Check sheet for the drawn part. Datum: minimum x, y, z corner. Units: mm. A direction names the side the tool comes from. Give positions to 0.01 mm unless a question says otherwise; leave off trailing zeros. Write each loop counter-clockwise with the first axis right and the second up, starting at its lowest first coordinate (ties: lowest second). Pieces come first, ordered by that corner, then holes. Notation, with made-up numbers: (87.5, 9.25) - (114.5, 9.25) arc R14 cw to (114.5, 26.25) - close; hole circle Ø3 at (49.25, 67.5). An arc over 180 degrees is marked (long way). One line per question, with ' | ' between items. Start each with the question number.
Q1. Section check B-B on z = 5. Record the boundary of the cut face in (x, y) (3 decimals), and give its area (3 significant figures).
Q2. Gauge pin test, flat ends, axial feed: P1, Ø6, axis at x = 6, y = 53.5, coming from the +Z side (3 decimals); P2, Ø3, axis at x = 7, y = 33, coming from the -Z side; P3, Ø2, axis at y = 25, z = 8, coming from the -X side. Record the tip position at first contact, or that the pin passes through.
Q3. Section check C-C on y = 53.4. Record the boundary of the cut face in (x, z) (3 decimals), and give its area (3 significant figures).
Q4. Set-up check for the marked faces 1 and 2: record each of +Z, -Z, +X, -X, +Y, -Y from which the full face is reachable in a straight line by a thin tool's end or side.
Q5. Section check A-A on x = 5. Record the boundary of the cut face in (y, z) (3 decimals).
Q6. Section check D-D on y = 31. Record the boundary of the cut face in (x, z) (3 decimals).
Q7. Thickness scan on L1, parallel to Y at x = 5, z = 3.7; L2, parallel to Y at x = 7, z = 0.5; L3, parallel to X at y = 40.5, z = 5 (3 decimals). Record the ranges inside material, lowest first. Write a range as [from, to].
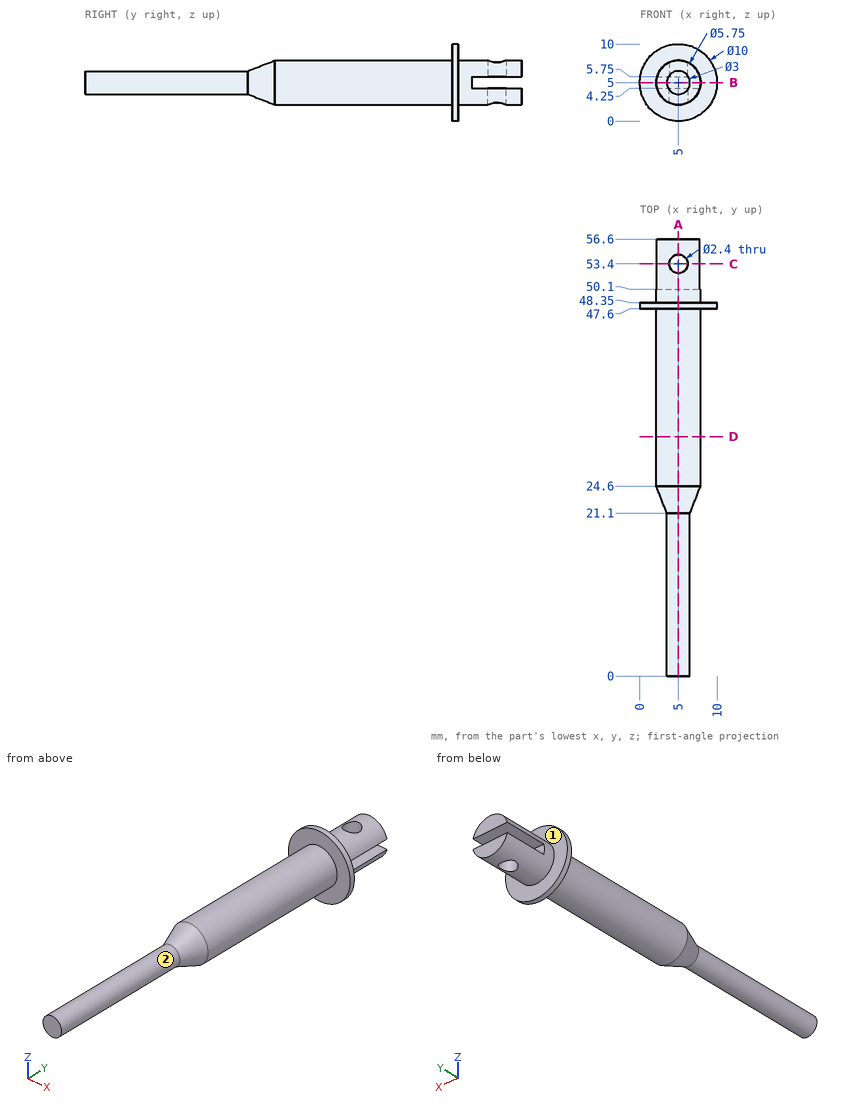
Working result:
1) outline: (0, 47.6) - (2.125, 47.6) - (2.125, 24.6) - (3.5, 21.1) - (3.5, 0) - (6.5, 0) - (6.5, 21.1) - (7.875, 24.6) - (7.875, 47.6) - (10, 47.6) - (10, 48.35) - (7.875, 48.35) - (7.875, 50.1) - (2.125, 50.1) - (2.125, 48.35) - (0, 48.35) - close | area: 228 mm2
2) P1: stops at z = 7.875 | P2: stops at z = 2.17 | P3: stops at x = 2.93
3) outline: (2.225, 4.25) arc R2.875 ccw to (3.8, 2.387) - (3.8, 4.25) - close; (2.225, 5.75) - (3.8, 5.75) - (3.8, 7.613) arc R2.875 ccw to start; (6.2, 2.387) arc R2.875 ccw to (7.775, 4.25) - (6.2, 4.25) - close; (6.2, 5.75) - (7.775, 5.75) arc R2.875 ccw to (6.2, 7.613) - close | area: 7.65 mm2
4) face 1: +Y | face 2: -Y
5) outline: (0, 3.5) - (21.1, 3.5) - (24.6, 2.125) - (47.6, 2.125) - (47.6, 0) - (48.35, 0) - (48.35, 2.125) - (52.2, 2.125) - (52.2, 4.25) - (50.1, 4.25) - (50.1, 5.75) - (52.2, 5.75) - (52.2, 7.875) - (48.35, 7.875) - (48.35, 10) - (47.6, 10) - (47.6, 7.875) - (24.6, 7.875) - (21.1, 6.5) - (0, 6.5) - close; (54.6, 2.125) - (56.6, 2.125) - (56.6, 4.25) - (54.6, 4.25) - close; (54.6, 5.75) - (56.6, 5.75) - (56.6, 7.875) - (54.6, 7.875) - close
6) outline: circle Ø5.75 at (5, 5)
7) L1: y = [0, 52.2], [54.6, 56.6] | L2: y = [47.6, 48.35] | L3: x = [2.125, 7.875]
